For this review, use the dimensioned drawing (mm, ordinates from the lowest corner) and the shaded views. A direction names the side the tool comes from. Give positions to 0.01 mm unless a question says otherwise; leave off trailing zeros. Loops run counter-clockwise (first coordinate to the right, second up) from the corner with the lowest first, then second, coordinate; pieces in that order, holes last. Notation, with made-up numbers: (-28.5, 31) - (-23.5, 31) arc R24 ccw to (-23.5, 46) - close; hole circle Ø10 at (60, -18). An arc over 180 degrees is marked (long way). Put each result on its own line as item: value.
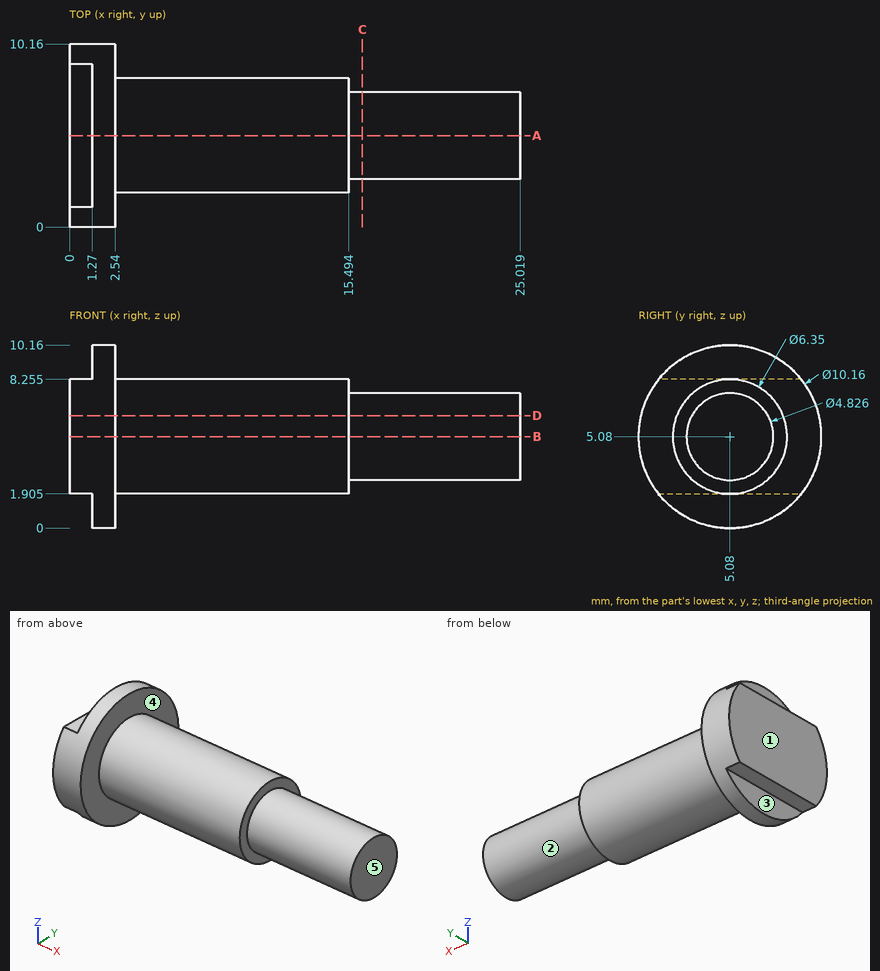
1) Draft analysis for pull direction Z (two halves, no side actions). For the marked faces 1 and 2, state which applies: pulls with the +Z half, pulls with the -Z half, needs draft (parallel to the pull), parting line crosses it, or undercut.
Geometry check:
face 1: needs draft
face 2: parting line crosses it
2) Take a section at D-D on z = 6.25. State the section outline as (x, y) points, and give its area (3 significant figures).
Geometry check:
outline: (0, 0.14) - (2.54, 0.14) - (2.54, 2.13) - (15.49, 2.13) - (15.49, 2.97) - (25.02, 2.97) - (25.02, 7.19) - (15.49, 7.19) - (15.49, 8.03) - (2.54, 8.03) - (2.54, 10.02) - (0, 10.02) - close
area: 142 mm²
3) Take a section at A-A on y = 5.08. State the section outline as (x, z) points (3 decimals), and give its area (3 significant figures).
Geometry check:
outline: (0, 1.905) - (1.27, 1.905) - (1.27, 0) - (2.54, 0) - (2.54, 1.905) - (15.494, 1.905) - (15.494, 2.667) - (25.019, 2.667) - (25.019, 7.493) - (15.494, 7.493) - (15.494, 8.255) - (2.54, 8.255) - (2.54, 10.16) - (1.27, 10.16) - (1.27, 8.255) - (0, 8.255) - close
area: 149 mm²
4) For the marked faces 3, 4 and 5, list the 3-axis set-ups (+Z, -Z, +X, -X, +Y, -Y) from which the entire face can be reached by the end or side of a thin tool; tool diameter is ignored.
Geometry check:
face 3: -Z, -X, +Y, -Y
face 4: +X
face 5: +Z, -Z, +X, +Y, -Y
5) Take a section at C-C on x = 16.25. State the section outline as (y, z) points.
Geometry check:
outline: circle Ø4.83 at (5.08, 5.08)
6) Wall thickness on line 1 (X direction, y = 4.75, z = 8.75); line 2 (Y direction, x = 2.5, z = 8.25); line 3 (X direction, y = 7.75, z = 6.5): over which ranges is each line inside the solid? List them lowest first.
Geometry check:
line 1: x = 1.27 to 2.54
line 2: y = 1.11 to 9.05
line 3: x = 0 to 15.49
7) Insertion check: pin 1 Ø2 at (y, z) = (5, 9.5) entering from -X; pin 2 Ø4 at (y, z) = (2.5, 7) entering from +X; pin 3 Ø6 at (x, z) = (22, 1.5) entering from -Y; pin 4 Ø0.6 at (x, y) = (0.5, 6) entering from +Z (3 decimals). Each pin has a flat end and moves straight along its axis. Give the tip position at first contact, or say it passes through.
Geometry check:
pin 1: stops at x = 1.27
pin 2: stops at x = 25.02
pin 3: stops at y = 2.74
pin 4: stops at z = 8.255
8) Take a section at B-B on z = 5.08. State the section outline as (x, y) points (3 decimals).
Geometry check:
outline: (0, 0) - (2.54, 0) - (2.54, 1.905) - (15.494, 1.905) - (15.494, 2.667) - (25.019, 2.667) - (25.019, 7.493) - (15.494, 7.493) - (15.494, 8.255) - (2.54, 8.255) - (2.54, 10.16) - (0, 10.16) - close
